from build123d import *

# Parameters (mm, degrees)
SKETCH1_W                     = 76.2
SKETCH1_H                     = 914.4
BOSS_EXTRUDE1_DEPTH           = 3.175
SKETCH2_W                     = 3.556
SKETCH2_H                     = 12.954
CUT_EXTRUDE1_DEPTH            = 4.175
LPATTERN1_COUNT               = 2
LPATTERN1_PITCH               = 50.8
LPATTERN1_COPY_1_SKETCH_W     = 3.556
LPATTERN1_COPY_1_SKETCH_H     = 12.954
LPATTERN1_COPY_1_DEPTH        = 4.175
LPATTERN1_COL_COUNT           = 2
LPATTERN1_COL_PITCH           = 50.8
LPATTERN1_COL_COPY_1_SKETCH_W = 3.556
LPATTERN1_COL_COPY_1_SKETCH_H = 12.954
LPATTERN1_COL_COPY_1_DEPTH    = 4.175
SKETCH3_W                     = 3.556
SKETCH3_H                     = 12.954
CUT_EXTRUDE2_DEPTH            = 4.175
F_8_CLEARANCE_HOLE1_D         = 4.4958
CUT_EXTRUDE3_DEPTH            = 1
CUT_EXTRUDE3_DEPTH_BACK       = 4.175
BOSS_EXTRUDE2_DEPTH           = 3.175
BOSS_EXTRUDE3_DEPTH           = 3.175
FILLET1_R                     = 25.4
F_8_CLEARANCE_HOLE2_D         = 4.4958


with BuildPart() as part:
    # Sketch1 → Boss-Extrude1 (new body)
    with BuildSketch(Plane(origin=(0, 0, 0), x_dir=(0, 0, -1), z_dir=(1, 0, 0))):
        Rectangle(SKETCH1_W, SKETCH1_H)
    extrude(amount=BOSS_EXTRUDE1_DEPTH)

    # Sketch2 → Cut-Extrude1 (cut, through all)
    with BuildSketch(Plane(origin=(3.175, 0, 0), x_dir=(0, 0, -1), z_dir=(1, 0, 0))):
        with Locations((5.499997, -211.0105)):
            Rectangle(SKETCH2_W, SKETCH2_H)
    cut_extrude1 = extrude(amount=-CUT_EXTRUDE1_DEPTH, mode=Mode.SUBTRACT)

    # Mirror1: Cut-Extrude1 across plane
    add(cut_extrude1.mirror(Plane.XY), mode=Mode.SUBTRACT)

    # LPattern1: Cut-Extrude1 ×2
    with Locations(*[(0, i * LPATTERN1_PITCH, 0) for i in range(1, LPATTERN1_COUNT)]):
        add(cut_extrude1, mode=Mode.SUBTRACT)

    # LPattern1 copy 1 sketch → LPattern1 copy 1 (cut, through all)
    with BuildSketch(Plane(origin=(3.175, 50.8, 0), x_dir=(0, 0, 1), z_dir=(1, 0, 0))):
        with Locations((5.499997, 211.0105)):
            Rectangle(LPATTERN1_COPY_1_SKETCH_W, LPATTERN1_COPY_1_SKETCH_H)
    extrude(amount=-LPATTERN1_COPY_1_DEPTH, mode=Mode.SUBTRACT)

    # LPattern1 col: Cut-Extrude1 ×2
    with Locations(*[(0, -i * LPATTERN1_COL_PITCH, 0) for i in range(1, LPATTERN1_COL_COUNT)]):
        add(cut_extrude1, mode=Mode.SUBTRACT)

    # LPattern1 col copy 1 sketch → LPattern1 col copy 1 (cut, through all)
    with BuildSketch(Plane(origin=(3.175, -50.8, 0), x_dir=(0, 0, 1), z_dir=(1, 0, 0))):
        with Locations((5.499997, 211.0105)):
            Rectangle(LPATTERN1_COL_COPY_1_SKETCH_W, LPATTERN1_COL_COPY_1_SKETCH_H)
    extrude(amount=-LPATTERN1_COL_COPY_1_DEPTH, mode=Mode.SUBTRACT)

    # Sketch3 → Cut-Extrude2 (cut, through all)
    with BuildSketch(Plane(origin=(3.175, 0, 0), x_dir=(0, 0, -1), z_dir=(1, 0, 0))):
        with Locations((5.499997, 164.431090402)):
            Rectangle(SKETCH3_W, SKETCH3_H)
        with Locations((-5.499997, 164.431090402)):
            Rectangle(SKETCH3_W, SKETCH3_H)
    extrude(amount=-CUT_EXTRUDE2_DEPTH, mode=Mode.SUBTRACT)

    # #8 Clearance Hole1 (through all)
    with Locations(Plane(origin=(3.175, 0, 0), x_dir=(0, 0, -1), z_dir=(1, 0, 0))):
        with Locations((6.35, -64.523692353), (-6.35, -64.523692353), (6.35, 81.271985669), (-6.35, 81.271985669), (5.25, -82.226052879), (-5.25, -82.226052879)):
            Hole(F_8_CLEARANCE_HOLE1_D / 2)

    # Sketch6 → Cut-Extrude3 (cut, two sides)
    with BuildSketch(Plane(origin=(3.175, 0, 0), x_dir=(0, 0, -1), z_dir=(1, 0, 0))) as cut_extrude3_sk:
        Polygon((-1346.127604676, 187.325), (-38.1, 187.325), (38.1, 187.325), (1346.127604676, 187.325), (1346.127604676, 2803.380209351), (-1346.127604676, 2803.380209351), align=None)
    extrude(amount=CUT_EXTRUDE3_DEPTH, mode=Mode.SUBTRACT)
    extrude(cut_extrude3_sk.sketch, amount=-CUT_EXTRUDE3_DEPTH_BACK, mode=Mode.SUBTRACT)

    # Sketch7 → Boss-Extrude2 (add)
    with BuildSketch(Plane(origin=(3.175, 0, 0), x_dir=(0, 0, -1), z_dir=(1, 0, 0))):
        Polygon((-38.1, -457.2), (-38.1, -501.65), (0, -501.65), (38.1, -501.65), (38.1, -457.2), align=None)
    extrude(amount=-BOSS_EXTRUDE2_DEPTH)

    # Sketch8 → Boss-Extrude3 (add)
    with BuildSketch(Plane(origin=(3.175, 0, 0), x_dir=(0, 0, -1), z_dir=(1, 0, 0))):
        Polygon((-38.1, -387.35), (-76.2, -476.25), (-76.2, -501.65), (76.2, -501.65), (76.2, -476.25), (38.1, -387.35), align=None)
    extrude(amount=-BOSS_EXTRUDE3_DEPTH)

    # Fillet1
    fillet1_edges = [part.edges().sort_by_distance(p)[0] for p in [
        (1.5875, -387.35, 38.1),
        (1.5875, -387.35, -38.1),
        (1.5875, -476.25, -76.2),
        (1.5875, -476.25, 76.2),
    ]]
    fillet(fillet1_edges, radius=FILLET1_R)

    # #8 Clearance Hole2 (through all)
    with Locations(Plane.ZY):
        with Locations((10.4775, 108.326326852), (-10.4775, 108.326326852), (-10.4775, 140.076326852), (10.4775, 140.076326852)):
            Hole(F_8_CLEARANCE_HOLE2_D / 2)


solid = part.part
Geometry check sheet. Reference: the model listing, model coordinates, mm. Give positions to 0.01 mm unless a question says otherwise; leave off trailing zeros. Order: outer loops, then holes, each group sorted by start corner. A loop starts at its lowest first (then second) coordinate and runs counter-clockwise, first axis right, second up.
1) Material ranges on probe 1 along Z at (x, y) = (1.8, 108.5); probe 2 along Z at (x, y) = (1, -326); probe 3 along Y at (x, z) = (2.25, -65.5), recorded low to high.
Results are:
probe 1: z = -38.1 to -12.72, -8.24 to 8.24, 12.72 to 38.1
probe 2: z = -38.1 to 38.1
probe 3: y = -501.65 to -451.28
2) Cross-section at C-C (x = 2). Give the number of separate pieces and of enclosed holes in the cut face, then the cut area to 3 significant figures.
Results are:
separate pieces: 1
enclosed holes: 18
area: 57,300 mm2
3) Cross-section at B-B (y = 119). Record the boundary of the cut face in (x, z) (3 decimals).
Results are:
outline: (0, -38.1) - (3.175, -38.1) - (3.175, 38.1) - (0, 38.1) - close
4) Cross-section at A-A (z = -57). Record the boundary of the cut face in (x, y) (3 decimals), then the cut area to 3 significant figures.
Results are:
outline: (0, -501.65) - (3.175, -501.65) - (3.175, -431.45) - (0, -431.45) - close
area: 223 mm2
5) Gauge pin test, flat ends, axial feed: pin 1 (1 mm diameter, centred on y = -302.5, z = 21.5, fed in from -X); pin 2 (1.6 mm diameter, centred on x = 1.5, y = -161.5, fed in from -Z). Record the tip position at first contact, or that the pin passes through.
Results are:
pin 1: stops at x = 0
pin 2: stops at z = -38.1
